Autodesk Inventor part; units mm, degrees
ref_plane "YZ Plane" through (0, 0, 0) normal (1, 0, 0) x (0, 1, 0)
ref_plane "XZ Plane" through (0, 0, 0) normal (0, 1, 0) x (-1, 0, 0)
ref_plane "XY Plane" through (0, 0, 0) normal (0, 0, 1) x (1, 0, 0)
sketch "Sketch1" plane through (0, 0, 0) normal (0, 1, 0) x (-1, 0, 0)
  circle A0 centre (0, 0) radius 8
  dimension "d0" = 16
extrude "Extrusion1" add sketch "Sketch1" along normal blind 8
sketch "Sketch2" plane through (0, 8, 0) normal (0, 1, 0) x (1, 0, 0)
  circle A0 centre (0, 0) radius 6
  dimension "d3" = 12
extrude "Extrusion2" add sketch "Sketch2" along normal blind 6
sketch "Sketch3" plane through (0, 14, 0) normal (0, 1, 0) x (1, 0, 0)
  circle A0 centre (0, 0) radius 8
  dimension "d6" = 16
extrude "Extrusion3" add sketch "Sketch3" along normal blind 1
sketch "Sketch4" plane through (0, 15, 0) normal (0, 1, 0) x (1, 0, 0)
  point P0 (0, 0)
  point P1 (0, 0)
hole "Hole1" at (0, 15, 0) direction (0, -1, 0) diameter 5 end through all
properties part number "GT2 20 Teeth Motor Pulley"
Can you work these out from the model? Positions are in its coordinate system, mm. A direction names the side the tool comes from. Give positions to 0.01 mm unless a question says otherwise; leave off trailing zeros. Order: outer loops, then holes, each group sorted by start corner. A loop starts at its lowest first (then second) coordinate and runs counter-clockwise, first axis right, second up. Notation, with made-up numbers: M 61.5,-36 L 69.5,-36 A35 ccw 69.5,-4 Z; hole C 55,70 d11. An arc over 180 degrees is marked long. One line per item, written item: value.
Item 1: If we section it at C-C on y = 1: Write out the boundary of the cut face in (x, z).
Verdict:
outline: C 0,0 d16; hole C 0,0 d5
Item 2: If we section it at B-B on x = 6.5: Write out the boundary of the cut face in (y, z).
Verdict:
outline: M 0,-4.66 L 8,-4.66 L 8,4.66 L 0,4.66 Z; M 14,-4.66 L 15,-4.66 L 15,4.66 L 14,4.66 Z
Item 3: Please list where these lines run through material, in increasing order: line 1 (Z direction, x = 0, y = 7); line 2 (Z direction, x = 0, y = 9.5).
Verdict:
line 1: -8 to -2.5, 2.5 to 8
line 2: -6 to -2.5, 2.5 to 6
Item 4: If we mould it in two halves opening along Y, with no side actions, what happens to faces 3 (the face through (-2, 14, -6)), 4 (the face through (-2, 15, 2)), 5 (the face through (2, 0, -2))? For each: pulls with the +Y half, pulls with the -Y half, needs draft (parallel to the pull), parting line crosses it, or undercut.
Verdict:
face 3: undercut
face 4: pulls with the +Y half
face 5: pulls with the -Y half
Item 5: If we section it at D-D on x = 0: Write out the boundary of the cut face in (y, z).
Verdict:
outline: M 0,-8 L 8,-8 L 8,-6 L 14,-6 L 14,-8 L 15,-8 L 15,-2.5 L 0,-2.5 Z; M 0,2.5 L 15,2.5 L 15,8 L 14,8 L 14,6 L 8,6 L 8,8 L 0,8 Z
Item 6: If we section it at A-A on z = 0: Write out the boundary of the cut face in (x, y).
Verdict:
outline: M -8,0 L -2.5,0 L -2.5,15 L -8,15 L -8,14 L -6,14 L -6,8 L -8,8 Z; M 2.5,0 L 8,0 L 8,8 L 6,8 L 6,14 L 8,14 L 8,15 L 2.5,15 Z
Item 7: For faces 1 (the face through (1.73, 3.94, 7.81)), 2 (the face through (-6, 11, 0)), which set-ups out of +Z, -Z, +X, -X, +Y, -Y let a thin tool reach every point of the face, with its end or its side?
Verdict:
face 1: +Y, -Y
face 2: none
Item 8: For pin 1 (8 mm diameter, centred on x = -4.5, y = 2.5, fed in from +Z); pin 2 (3 mm diameter, centred on x = 4.5, y = 11, fed in from -Z); pin 3 (1 mm diameter, centred on x = -1, y = 11, fed in from -Z), each with a flat end and sliding along its axis, tell me the tip position at first contact or that it passes through.
Verdict:
pin 1: z = 7.98
pin 2: z = -5.2
pin 3: z = -5.98
